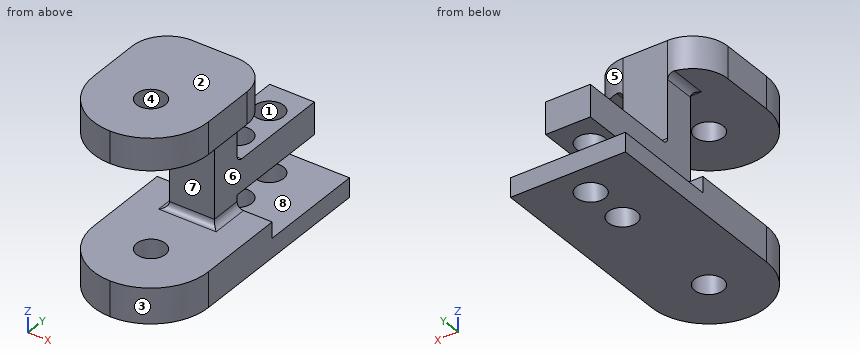
```python
from build123d import *

# Parameters (mm, degrees)
ESQUISSE1_W             = 20
ESQUISSE1_H             = 17
ESQUISSE1_R             = 2.1
BOSS_EXTRU_1_DEPTH      = 5
ESQUISSE2_W             = 18
ESQUISSE2_H             = 3
BOSS_EXTRU_3_DEPTH      = 23
ESQUISSE5_W             = 6.5
ESQUISSE5_H             = 17
ENL_V_MAT_EXTRU_3_DEPTH = 18
ESQUISSE10_W            = 7
ESQUISSE10_H            = 3
BOSS_EXTRU_6_DEPTH      = 10
ESQUISSE11_W            = 5.5
ESQUISSE11_H            = 2.5
ESQUISSE11_W_2          = 7
ESQUISSE11_H_2          = 0.5
BOSS_EXTRU_7_DEPTH      = 17
ESQUISSE12_W            = 18
ESQUISSE12_H            = 2.5
BOSS_EXTRU_8_DEPTH      = 23
CONG_3_R                = 9
ESQUISSE20_R            = 2.25
ENL_V_MAT_EXTRU_7_DEPTH = 18
ESQUISSE22_W            = 7
ESQUISSE22_H            = 5
BOSS_EXTRU_9_DEPTH      = 23
ESQUISSE27_W            = 5.5
ESQUISSE27_H            = 5
ESQUISSE27_W_2          = 7
BOSS_EXTRU_10_DEPTH     = 23
CONG_4_R                = 9
ESQUISSE28_R            = 2.25
ENL_V_MAT_EXTRU_8_DEPTH = 44
CONG_5_R                = 1
CONG_6_R                = 5.5


with BuildPart() as part:
    # Esquisse1 → Boss.-Extru.1 (new body)
    with BuildSketch(Plane.XY):
        with Locations((10, 8.5)):
            Rectangle(ESQUISSE1_W, ESQUISSE1_H)
        with Locations((10, 5)):
            Circle(ESQUISSE1_R, mode=Mode.SUBTRACT)
        with Locations((10, 12)):
            Circle(ESQUISSE1_R, mode=Mode.SUBTRACT)
    extrude(amount=BOSS_EXTRU_1_DEPTH)

    # Esquisse5 → Enlèv. mat.-Extru.3 (cut)
    with BuildSketch(Plane.XY.offset(5)):
        with Locations((16.75, 8.5)):
            Rectangle(ESQUISSE5_W, ESQUISSE5_H)
        with Locations((3.25, 8.5)):
            Rectangle(ESQUISSE5_W, ESQUISSE5_H)
    extrude(amount=-ENL_V_MAT_EXTRU_3_DEPTH, mode=Mode.SUBTRACT)



with BuildPart() as body_2:
    # Esquisse2 → Boss.-Extru.3 (new body)
    with BuildSketch(Plane.XZ):
        with Locations((10, -3.5)):
            Rectangle(ESQUISSE2_W, ESQUISSE2_H)
    extrude(amount=BOSS_EXTRU_3_DEPTH)


with BuildPart() as part_1:
    add(part.part)

    add(body_2.part)  # Boss.-Extru.6 merges body 2
    # Esquisse10 → Boss.-Extru.6 (add)
    with BuildSketch(Plane.XY.offset(5)):
        with Locations((10, -1.5)):
            Rectangle(ESQUISSE10_W, ESQUISSE10_H)
    extrude(amount=-BOSS_EXTRU_6_DEPTH)

    # Esquisse11 → Boss.-Extru.7 (add)
    with BuildSketch(Plane(origin=(0, 0, 0), x_dir=(1, 0, 0), z_dir=(0, 1, 0))):
        with Locations((3.75, 6.25)):
            Rectangle(ESQUISSE11_W, ESQUISSE11_H)
        with Locations((10, 6.25)):
            Rectangle(ESQUISSE11_W_2, ESQUISSE11_H)
        with Locations((16.25, 6.25)):
            Rectangle(ESQUISSE11_W, ESQUISSE11_H)
        with Locations((3.75, 4.75)):
            Rectangle(ESQUISSE11_W, ESQUISSE11_H_2)
        with Locations((10, 4.75)):
            Rectangle(ESQUISSE11_W_2, ESQUISSE11_H_2)
        with Locations((16.25, 4.75)):
            Rectangle(ESQUISSE11_W, ESQUISSE11_H_2)
    extrude(amount=BOSS_EXTRU_7_DEPTH)

    # Esquisse12 → Boss.-Extru.8 (add)
    with BuildSketch(Plane.XZ):
        with Locations((10, -6.25)):
            Rectangle(ESQUISSE12_W, ESQUISSE12_H)
    extrude(amount=BOSS_EXTRU_8_DEPTH)

    # Congé3
    cong_3_edges = [part_1.edges().sort_by_distance(p)[0] for p in [
        (19, -23, -4.75),
        (1, -23, -4.75),
    ]]
    fillet(cong_3_edges, radius=CONG_3_R - 0.0001)  # a hair under: the kernel refuses the full size

    # Esquisse20 → Enlèv. mat.-Extru.7 (cut)
    with BuildSketch(Plane.XY.offset(5)):
        with Locations((10, 5)):
            Circle(ESQUISSE20_R)
        with Locations((10, 12)):
            Circle(ESQUISSE20_R)
    extrude(amount=-ENL_V_MAT_EXTRU_7_DEPTH, mode=Mode.SUBTRACT)

    # Esquisse22 → Boss.-Extru.9 (add)
    with BuildSketch(Plane.XY.offset(-2)):
        with Locations((10, -2.5)):
            Rectangle(ESQUISSE22_W, ESQUISSE22_H)
    extrude(amount=BOSS_EXTRU_9_DEPTH)

    # Esquisse27 → Boss.-Extru.10 (add)
    with BuildSketch(Plane(origin=(0, 0, 0), x_dir=(1, 0, 0), z_dir=(0, 1, 0))):
        with Locations((3.75, -18.5)):
            Rectangle(ESQUISSE27_W, ESQUISSE27_H)
        with Locations((16.25, -18.5)):
            Rectangle(ESQUISSE27_W, ESQUISSE27_H)
        with Locations((10, -18.5)):
            Rectangle(ESQUISSE27_W_2, ESQUISSE27_H)
    extrude(amount=-BOSS_EXTRU_10_DEPTH)

    # Congé4
    cong_4_edges = [part_1.edges().sort_by_distance(p)[0] for p in [
        (1, -23, 18.5),
        (19, -23, 18.5),
    ]]
    fillet(cong_4_edges, radius=CONG_4_R - 0.0001)  # a hair under: the kernel refuses the full size

    # Esquisse28 → Enlèv. mat.-Extru.8 (cut)
    with BuildSketch(Plane.XY.offset(21)):
        with Locations((10, -14)):
            Circle(ESQUISSE28_R)
    extrude(amount=-ENL_V_MAT_EXTRU_8_DEPTH, mode=Mode.SUBTRACT)

    # Congé5
    cong_5_edges = [part_1.edges().sort_by_distance(p)[0] for p in [
        (10, 0, 5),
        (10, -5, -2),
        (10, -5, 16),
        (6.5, -2.5, 16),
        (13.5, -2.5, 16),
        (6.5, -2.5, -2),
        (13.5, -2.5, -2),
    ]]
    fillet(cong_5_edges, radius=CONG_5_R)

    # Congé6
    cong_6_edges = [part_1.edges().sort_by_distance(p)[0] for p in [
        (1, 0, 18.5),
        (19, 0, 18.5),
    ]]
    fillet(cong_6_edges, radius=CONG_6_R - 0.0001)  # a hair under: the kernel refuses the full size


solid = part_1.part
```
Read the model definition and answer for the solid it produces. Units are mm, in the model's axes. Face numbers are marked on the shaded views. A direction names the side the tool comes from. Give positions to 0.01 mm unless a question says otherwise; leave off trailing zeros. Write each loop counter-clockwise with the first axis right and the second up, starting at its lowest first coordinate (ties: lowest second). Pieces come first, ordered by that corner, then holes. Notation, with made-up numbers: (82.5, 57.25) -> (107.5, 57.25) arc R26 cw to (107.5, 87.25) -> close; hole circle Ø11 at (30, 3). An arc over 180 degrees is marked (long way). Answer in a Markdown table with one row per item.
1) Section C-C on x = 5 is taken. Give the vertices of the cut face in (y, z).
Results list:
| item | result |
|---|---|
| outline | (-21.48, -7.5) -> (17, -7.5) -> (17, -4.5) -> (0, -4.5) -> (0, -2) -> (-21.48, -2) -> close; (-21.48, 16) -> (-0.21, 16) -> (-0.21, 21) -> (-21.48, 21) -> close |
2) Section B-B on y = -8 is taken. Give the vertices of the cut face in (x, z).
Results list:
| item | result |
|---|---|
| outline | (1, -7.5) -> (19, -7.5) -> (19, -2) -> (1, -2) -> close; (1, 16) -> (19, 16) -> (19, 21) -> (1, 21) -> close |
3) Section D-D on z = 9.75 is taken. Give the vertices of the cut face in (x, y).
Results list:
| item | result |
|---|---|
| outline | (6.5, -5) -> (13.5, -5) -> (13.5, 0) -> (6.5, 0) -> close |
4) Each of these flat-tipped pins is pushed along its axis until it touches: pin 1 Ø5.5 at (x, z) = (10, 17) entering from +Y; pin 2 Ø4 at (x, y) = (10, 5) entering from -Z; pin 3 Ø2 at (x, y) = (11.5, 10.5) entering from +Z; pin 4 Ø10 at (y, z) = (9, 9) entering from +X. Where does it stop, or does it pass through?
Results list:
| item | result |
|---|---|
| pin 1 | y = 0 |
| pin 2 | through |
| pin 3 | z = 5 |
| pin 4 | x = 13.5 |
5) Determine the mould class of the marked faces 1, 2, 3 and 4 for opening direction X: released by +X, released by -X, zero draft, split by the parting line, or undercut.
Results list:
| item | result |
|---|---|
| face 1 | undercut |
| face 2 | zero draft |
| face 3 | released by +X |
| face 4 | undercut |
6) A tool of negligible diameter and unlimited length cuts with its end or side. For the marked faces 5, 6, 7 and 8, from which of +Z, -Z, +X, -X, +Y, -Y can it reach the whole face along a straight path? Write none if from no direction.
Results list:
| item | result |
|---|---|
| face 5 | +Z, +X, +Y |
| face 6 | +X, +Y, -Y |
| face 7 | +X, -X, -Y |
| face 8 | +X, -X, +Y |
7) Section A-A on y = 5 is taken. Give the vertices of the cut face in (x, z).
Results list:
| item | result |
|---|---|
| outline | (1, -7.5) -> (7.75, -7.5) -> (7.75, -4.5) -> (1, -4.5) -> close; (6.5, 0) -> (7.75, 0) -> (7.75, 5) -> (6.5, 5) -> close; (12.25, -7.5) -> (19, -7.5) -> (19, -4.5) -> (12.25, -4.5) -> close; (12.25, 0) -> (13.5, 0) -> (13.5, 5) -> (12.25, 5) -> close |
8) Straight lines are drawn through the part: line 1 (Y direction, x = 10, z = 3.9); line 2 (Z direction, x = 10, y = 14.5); line 3 (Z direction, x = 10.75, y = -9). For each, find the intervals that lie inside material, in ascending order. Write a range as [from, to].
Results list:
| item | result |
|---|---|
| line 1 | [-5, 2.75], [7.25, 9.75], [14.25, 17] |
| line 2 | [-7.5, -4.5], [0, 5] |
| line 3 | [-7.5, -2], [16, 21] |
